Design review of the part built by this model. Coordinates are the model's own, in mm. Round coordinates to 2 decimals unless told otherwise and drop trailing zeros. Loops run counter-clockwise (first coordinate to the right, second up) from the corner with the lowest first, then second, coordinate; pieces in that order, holes last. Notation, with made-up numbers: (42.5, 14.25) - (74.5, 14.25) arc R25 cw to (74.5, 36.25) - close; hole circle Ø9 at (30, 63.25). An arc over 180 degrees is marked (long way). Use one line per item in the form item = value. Start each with the question number.
(1) Wall thickness on probe 1 along X at (y, z) = (-2, 135); probe 2 along X at (y, z) = (-1, 99); probe 3 along Y at (x, z) = (-4, 191): over which ranges is each line inside the solid? List them lowest first. Write a range as [from, to].
(2) We need section A-A, the plane z = 17. Write out the cut boundary in (x, y).
(3) For pin 1 (4 mm diameter, centred on y = -3, z = -172, fed in from +X), flat-tipped, find the tip position at first contact; note if it passes through.
Autodesk Inventor part; units mm, degrees
ref_plane "YZ Plane" through (0, 0, 0) normal (1, 0, 0) x (0, 1, 0)
ref_plane "XZ Plane" through (0, 0, 0) normal (0, 1, 0) x (-1, 0, 0)
ref_plane "XY Plane" through (0, 0, 0) normal (0, 0, 1) x (1, 0, 0)
sketch "草图1" plane through (0, 0, 0) normal (0, 0, 1) x (1, 0, 0)
  circle A0 centre (0, 0) radius 5
  dimension "d0" = 10
extrude "拉伸1" add sketch "草图1" along normal mid plane 530
sketch "草图2" plane through (0, 0, 0) normal (0, 1, 0) x (-1, 0, 0)
  arc A0 (4.5149, 268.9403) -> (5, 265) centre (5, 267) ccw
  line L0 (5, 265) -> (-5, 265)
  line L1 (3, 275) -> (4.5149, 268.9403)
  line L2 (3, 275) -> (0, 275)
  line L3 (0, 275) -> (0, 265)
  line L4 (5, 265) -> (0, 265)
  point P0 (0, 0)
  dimension "d4" = 2
  dimension "d5" = 2
  dimension "d7" = 10
  dimension "d10" = 5
  dimension "d11" = 3
revolve "旋转1" add sketch "草图2" angle 360 about axis through (0, 0, 275) along (0, 0, -1)
mirror "镜像1" about plane through (0, 0, 0) normal (0, 0, 1) of "旋转1"
properties part number "载板连接销"
Data:
q1.probe_1 = [-4.58, 4.58]
q1.probe_2 = [-4.9, 4.9]
q1.probe_3 = [-3, 3]
q2.outline = circle Ø10 at (0, 0)
q3.pin_1 = 4.9
